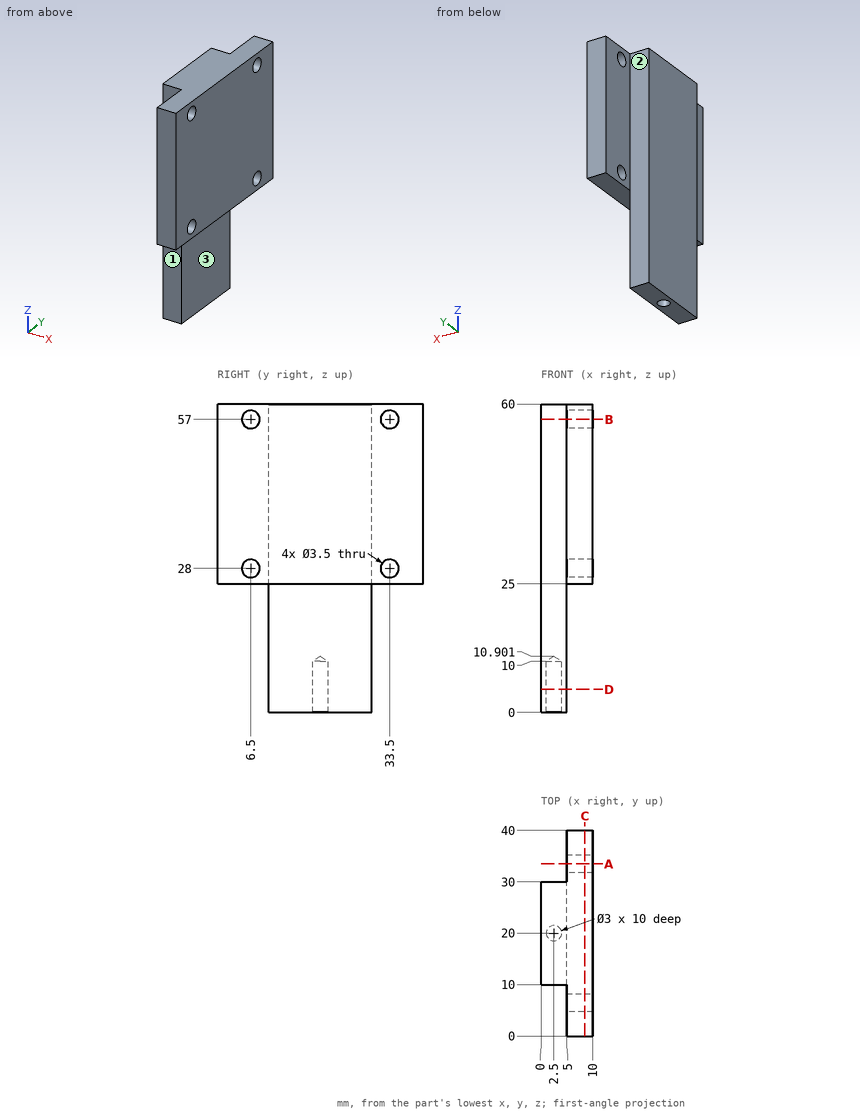
Answer from the drawing. Dimensions are ordinates in mm from the lowest x, y and z of the part. A direction names the side the tool comes from. Round coordinates to 2 decimals unless told otherwise and drop trailing zeros. Write each loop counter-clockwise with the first axis right and the second up, starting at its lowest first coordinate (ties: lowest second). Pieces come first, ordered by that corner, then holes. Notation, with made-up numbers: M 29,73.25 L 60,73.25 A32 cw 60,111.25 Z; hole C 24,58 d10. An arc over 180 degrees is marked long. Write each question's results on one line, items separated by ' | '. Start each with the question number.
Item 1: Find section B-B on z = 57. Write down the section's boundary in (x, y), and give its area (3 significant figures).
Item 2: Find section D-D on z = 4.5. Write down the section's boundary in (x, y).
Item 3: Find section A-A on y = 33.5. Write down the section's boundary in (x, z).
Item 4: Find section C-C on x = 8.5. Write down the section's boundary in (y, z).
Item 5: Straight lines are drawn through the part: probe 1 along Z at (x, y) = (6.2, 6.5); probe 2 along X at (y, z) = (20, 6.5); probe 3 along Z at (x, y) = (7.5, 8). For each, find the intervals that lie inside material, in ascending order.
Item 6: Given pin 1 Ø5 at (y, z) = (5, 34) entering from -X; pin 2 Ø1.5 at (x, z) = (1.5, 41.5) entering from +Y; pin 3 Ø22 at (y, z) = (20, 7.5) entering from +X; pin 4 Ø4 at (x, z) = (7.5, 8) entering from -Y, each flat-ended and moving along its own axis, determine where each tip first touches the part or whether it passes through.
Item 7: Which of the six approach directions +Z, -Z, +X, -X, +Y, -Y give full straight-line access (tool end or side, diameter ignored) to the marked faces 1, 2 and 3?
Answer block:
1) outline: M 0,10 L 5,10 L 5,8.25 L 10,8.25 L 10,31.75 L 5,31.75 L 5,30 L 0,30 Z; M 5,0 L 10,0 L 10,4.75 L 5,4.75 Z; M 5,35.25 L 10,35.25 L 10,40 L 5,40 Z | area: 265 mm²
2) outline: M 0,10 L 5,10 L 5,30 L 0,30 Z; hole C 2.5,20 d3
3) outline: M 5,25 L 10,25 L 10,26.25 L 5,26.25 Z; M 5,29.75 L 10,29.75 L 10,55.25 L 5,55.25 Z; M 5,58.75 L 10,58.75 L 10,60 L 5,60 Z
4) outline: M 0,25 L 40,25 L 40,60 L 0,60 Z; hole C 6.5,28 d3.5; hole C 6.5,57 d3.5; hole C 33.5,28 d3.5; hole C 33.5,57 d3.5
5) probe 1: z = 25 to 26.25, 29.75 to 55.25, 58.75 to 60 | probe 2: x = 0 to 1, 4 to 5 | probe 3: z = 25 to 27.1, 28.9 to 56.1, 57.9 to 60
6) pin 1: stops at x = 5 | pin 2: stops at y = 30 | pin 3: stops at x = 5 | pin 4: passes through
7) face 1: +Z, -Z, -X, -Y | face 2: +Z, -Z, -X, +Y | face 3: -Z, +X, +Y, -Y
